from build123d import *

# Parameters (mm, degrees)
F1_DEPTH = 2
F2_R     = 50
F3_SIZE2 = 0.57734
F3_SIZE  = 0.99999


# Not quite as in the source:
# - a fillet or chamfer is up to 0.001 mm smaller than in the source, because OpenCascade refuses the exact size


with BuildPart() as f1:
    # F0 (on Front) → F1 (new body)
    with BuildSketch(Plane.XZ):
        Polygon((0, 55), (0, 0), (38.8908729653, -38.8908729653), (25.2356788824, 29.7643211176), align=None)
    extrude(amount=F1_DEPTH)

    # F2
    f2_edges = [f1.edges().sort_by_distance(p)[0] for p in [
        (25.235679, -1, 29.764321),
    ]]
    fillet(f2_edges, radius=F2_R)

    # F3 (size 1 and 0.5773502692 in the source; OpenCascade refuses exactly that, so slightly less here)
    f3_edges = [f1.edges().sort_by_distance(p)[0] for p in [
        (7.255218, -2, 47.744782),
        (7.255218, 0, 47.744782),
    ]]
    f3_side = f1.faces().sort_by_distance((7.255218, -1, 47.744782))[0]
    chamfer(f3_edges, length=F3_SIZE, length2=F3_SIZE2, reference=f3_side)


solid = f1.part
The model under review builds one solid part; all positions refer to its coordinate system, in mm. Round coordinates to 2 decimals unless told otherwise and drop trailing zeros. Order: outer loops, then holes, each group sorted by start corner. A loop starts at its lowest first (then second) coordinate and runs counter-clockwise, first axis right, second up. Notation, with made-up numbers: (-26, 2) -> (-2, 2) arc R31 cw to (-2, 26) -> close; hole circle Ø11 at (40.25, 0.25). An arc over 180 degrees is marked (long way). Write item = value, one per line. Start each with the question number.
Item 1: Clearance check with a flat-ended pin moving along its axis: pin 1 Ø8 at (x, z) = (6, 9.5) entering from +Y. State where the tip first meets the part, or that it passes through.
Item 2: For line 1 along Z through (x, y) = (25, -0.45); line 2 along Z through (x, y) = (14, -1.5); line 3 along X through (y, z) = (-0.85, 4), list the stretches that pass through material, from the lowest coordinate up.
Item 3: Consider section C-C on y = -1.5. Write out the cut boundary in (x, z), plus the area to 3 significant figures.
Conclusion:
q1.pin_1 = 0
q2.line_1 = -25 to 24.28
q2.line_2 = -14 to 40.59
q2.line_3 = 0 to 30.27
q3.outline = (0, 0) -> (38.52, -38.52) -> (27.91, 14.83) arc R49.71 ccw to (14.31, 40.29) -> (0, 54.59) -> close
q3.area = 1,710 mm2
